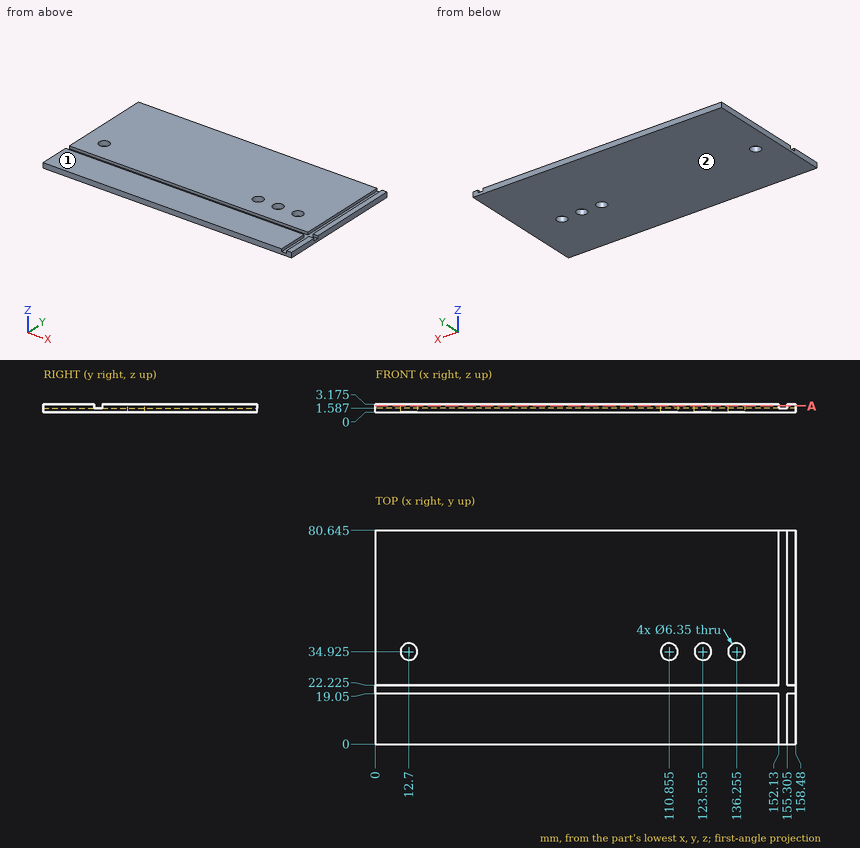
Study the drawing (mm; zero at the part's minimum x, y, z) and answer. Give positions to 0.01 mm unless a question says otherwise; leave off trailing zeros. One line per item, written item: value.
1. Each of these flat-tipped pins is pushed along its axis until it touches: P1, Ø3, axis at x = 62.5, y = 21.5, coming from the -Z side; P2, Ø5, axis at x = 136.255, y = 34.925, coming from the -Z side. Where does it stop, or does it pass through?
Found:
P1: z = 0
P2: through
2. Find the intervals of material crossed by probe 1 along X at (y, z) = (64, 1.8) (1 decimal); probe 2 along X at (y, z) = (36, 2.5) (1 decimal); probe 3 along Z at (x, y) = (84, 21.5), in increasing order.
Found:
probe 1: 0 to 152.1, 155.3 to 158.5
probe 2: 0 to 9.7, 15.7 to 107.9, 113.8 to 120.6, 126.5 to 133.3, 139.2 to 152.1, 155.3 to 158.5
probe 3: 0 to 1.59
3. For a pull along Z with two mould halves and no side action, classify the marked faces 1 and 2 as pulls with the +Z half, pulls with the -Z half, needs draft (parallel to the pull), parting line crosses it, or undercut.
Found:
face 1: pulls with the +Z half
face 2: pulls with the -Z half
4. Section A-A on z = 2.45 is taken. State how many separate pieces and enclosed holes the cut face has, plus the area to 3 significant figures.
Found:
separate pieces: 4
enclosed holes: 4
area: 11,900 mm^2
